from build123d import *

# Parameters (mm, degrees)
F1_DEPTH = 9
F2_T     = -1
F3_W     = 13
F3_H     = 5.063144
F4_DEPTH = 8.9
F5_W     = 35.64187
F5_H     = 5.863439
F6_DEPTH = 9.9
F7_W     = 41.68
F7_H     = 6.419253
F8_DEPTH = 25


with BuildPart() as f1:
    # F0 (on Top) → F1 (new body)
    with BuildSketch(Plane.XY):
        with BuildLine():
            ThreePointArc((31, 52.84), (28.024205, 60.024205), (20.84, 63))
            Line((20.84, 63), (-20.84, 63))
            ThreePointArc((-20.84, 63), (-28.024205, 60.024205), (-31, 52.84))
            Line((-31, 52.84), (-31, -52.84))
            ThreePointArc((-31, -52.84), (-28.024205, -60.024205), (-20.84, -63))
            Line((-20.84, -63), (20.84, -63))
            ThreePointArc((20.84, -63), (28.024205, -60.024205), (31, -52.84))
            Line((31, -52.84), (31, 52.84))
        make_face()
    extrude(amount=F1_DEPTH)

    # F2
    f2_openings = [f1.faces().sort_by_distance(p)[0] for p in [
        (0, 0, 9),
    ]]
    offset(amount=F2_T, openings=f2_openings)

    # F3 (on face) → F4 (cut)
    with BuildSketch(Plane(origin=(0, 63, 0), x_dir=(-1, 0, 0), z_dir=(0, 1, 0))):
        with Locations((-14.212146, 4.273678)):
            Rectangle(F3_W, F3_H)
    extrude(amount=-F4_DEPTH, mode=Mode.SUBTRACT)

    # F5 (on face) → F6 (cut)
    with BuildSketch(Plane(origin=(-31, 0, 0), x_dir=(0, -1, 0), z_dir=(-1, 0, 0))):
        with Locations((-32.919836, 4.599208)):
            Rectangle(F5_W, F5_H)
    extrude(amount=-F6_DEPTH, mode=Mode.SUBTRACT)

    # F7 (on face) → F8 (cut)
    with BuildSketch(Plane.XZ.offset(63)):
        with Locations((0, 4.608059)):
            Rectangle(F7_W, F7_H)
    extrude(amount=-F8_DEPTH, mode=Mode.SUBTRACT)


solid = f1.part
The listing builds one solid part. Answer for the finished solid, in the listing's coordinates (mm). A direction names the side the tool comes from. Round coordinates to 2 decimals unless told otherwise and drop trailing zeros. Order: outer loops, then holes, each group sorted by start corner. A loop starts at its lowest first (then second) coordinate and runs counter-clockwise, first axis right, second up. Notation, with made-up numbers: (33.5, 13.5) -> (79.5, 13.5) arc R28 cw to (79.5, 52.5) -> close; hole circle Ø7 at (14, 9). An arc over 180 degrees is marked (long way). One line per item, written item: value.
Item 1: For a pull along X with two mould halves and no side action, classify faces 1 (the cylindrical face through (-27.245, 59.388, 4.944)), 2 (the cylindrical face through (-27.945, 60.103, 4.437)), 3 (the flat face through (0, 1, 0)), 4 (the cylindrical face through (28.103, 59.945, 4.437)) as released by +X, released by -X, zero draft, split by the parting line, or undercut.
Taken from the geometry:
face 1: undercut
face 2: released by -X
face 3: zero draft
face 4: released by +X
Item 2: Find section C-C, the plane x = 19. Give the vertices of the cut face in (y, z), then the cut area to 3 significant figures.
Taken from the geometry:
outline: (-63, 0) -> (63, 0) -> (63, 1.74) -> (62, 1.74) -> (62, 1) -> (-62, 1) -> (-62, 1.4) -> (-63, 1.4) -> close; (-63, 7.82) -> (-62, 7.82) -> (-62, 9) -> (-63, 9) -> close; (62, 6.81) -> (63, 6.81) -> (63, 9) -> (62, 9) -> close
area: 131 mm2
Item 3: For faces 5 (the flat face through (-31, -11, 4)), 6 (the flat face through (30, -1, 5)), determine the directions among +Z, -Z, +X, -X, +Y, -Y from which every point of the face is accessible in a straight line to the end or side of a thin tool.
Taken from the geometry:
face 5: +Z, -Z, -X, +Y, -Y
face 6: +Z
Item 4: Find section D-D, the plane z = 3.5. Give the vertices of the cut face in (x, y), then the cut area to 3 significant figures.
Taken from the geometry:
outline: (-31, -52.84) arc R10.16 ccw to (-20.84, -63) -> (-20.84, -62) arc R9.16 cw to (-30, -52.84) -> (-30, 15.1) -> (-31, 15.1) -> close; (-31, 50.74) -> (-30, 50.74) -> (-30, 52.84) arc R9.16 cw to (-20.84, 62) -> (7.71, 62) -> (7.71, 63) -> (-20.84, 63) arc R10.16 ccw to (-31, 52.84) -> close; (20.71, 62) -> (20.84, 62) arc R9.16 cw to (30, 52.84) -> (30, -52.84) arc R9.16 cw to (20.84, -62) -> (20.84, -63) arc R10.16 ccw to (31, -52.84) -> (31, 52.84) arc R10.16 ccw to (20.84, 63) -> (20.71, 63) -> close
area: 265 mm2
Item 5: Find section A-A, the plane x = -6. Give the vertices of the cut face in (y, z), then the cut area to 3 significant figures.
Taken from the geometry:
outline: (-63, 0) -> (63, 0) -> (63, 9) -> (62, 9) -> (62, 1) -> (-62, 1) -> (-62, 1.4) -> (-63, 1.4) -> close; (-63, 7.82) -> (-62, 7.82) -> (-62, 9) -> (-63, 9) -> close
area: 136 mm2
Item 6: Find section B-B, the plane y = 27. Give the vertices of the cut face in (x, z).
Taken from the geometry:
outline: (-31, 0) -> (31, 0) -> (31, 9) -> (30, 9) -> (30, 1) -> (-30, 1) -> (-30, 1.67) -> (-31, 1.67) -> close; (-31, 7.53) -> (-30, 7.53) -> (-30, 9) -> (-31, 9) -> close
Item 7: Given P1, Ø1.5, axis at x = -3.5, y = -42, coming from the +Z side; P2, Ø4, axis at x = 24.5, z = 2.5, coming from the -Y side; P3, Ø0.5, axis at x = -30.5, z = 4.5, coming from the +Y side, each flat-ended and moving along its own axis, determine where each tip first touches the part or whether it passes through.
Taken from the geometry:
P1: stops at z = 1
P2: stops at y = -62.86
P3: stops at y = 56.67
Item 8: Straight lines are drawn through the part: L1, parallel to X at y = 13, z = 6; L2, parallel to Y at x = -4, z = 8; L3, parallel to Z at x = 8.5, y = -40. For each, find the intervals that lie inside material, in ascending order.
Taken from the geometry:
L1: x = -31 to -30, 30 to 31
L2: y = -63 to -62, 62 to 63
L3: z = 0 to 1
